Build history of the part. All positions in model axes, mm. Face numbers are marked on the shaded views. A direction names the side the tool comes from. Give positions to 0.01 mm unless a question says otherwise; leave off trailing zeros. Write each loop counter-clockwise with the first axis right and the second up, starting at its lowest first coordinate (ties: lowest second). Pieces come first, ordered by that corner, then holes. Notation, with made-up numbers: (-17, 12.5) -> (-3, 12.5) arc R13 ccw to (-3, 28.5) -> close; hole circle Ø7 at (19.5, 12.5). An arc over 180 degrees is marked (long way). Write item = value, one per line. Start each with the question number.
Q1. Saw through at C-C, the plane z = 5. List the corners of the cut face in (x, y), then the cut area to 3 significant figures.
Q2. Tool access for the marked faces 1 and 2: list every direction of +Z, -Z, +X, -X, +Y, -Y with a clear straight run to the whole face (end or side of a thin tool).
Q3. Saw through at B-B, the plane x = -2.5. List the corners of the cut face in (y, z).
Q4. Wall check: line 1 (Z direction, x = -3.5, y = -0.5); line 2 (X direction, y = -1.5, z = 7.75); line 3 (X direction, y = 5, z = 11.5). Give the ranges that are in metal, low to high.
Q5. Drop flat-ended pins along their axis: P1, Ø8, axis at x = -2, z = 7.5, coming from the +Y side; P2, Ø5, axis at y = 2, z = 6.5, coming from the -X side; P3, Ø5.5, axis at y = 3, z = 9.5, coming from the -X side; P4, Ø5.5, axis at y = 2, z = 9.5, coming from the +X side. Give the stop position or say it passes through.
Q6. Saw through at D-D, the plane x = 5.75. List the corners of the cut face in (y, z), then the cut area to 3 significant figures.
Q7. Mould opens along Y. For the marked faces 3, 4, 5 and 6 say: pulls with the +Y half, pulls with the -Y half, needs draft (parallel to the pull), parting line crosses it, or undercut.
Q8. Saw through at A-A, the plane y = 2. List the corners of the cut face in (x, z), then the cut area to 3 significant figures.
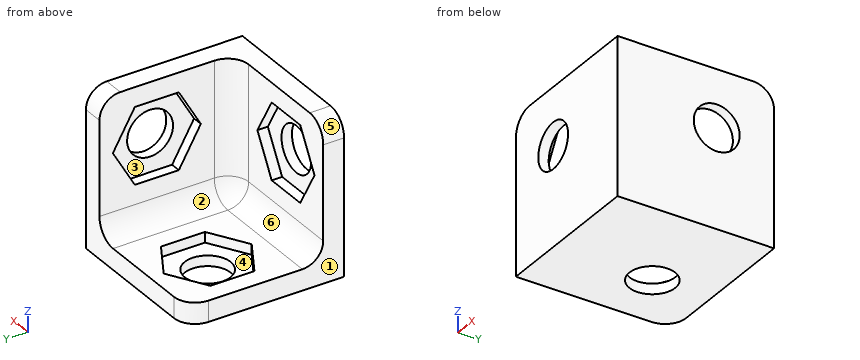
Autodesk Inventor part; units mm, degrees
ref_plane "YZ Plane" through (0, 0, 0) normal (1, 0, 0) x (0, 1, 0)
ref_plane "XZ Plane" through (0, 0, 0) normal (0, 1, 0) x (-1, 0, 0)
ref_plane "XY Plane" through (0, 0, 0) normal (0, 0, 1) x (1, 0, 0)
sketch "Sketch1" plane through (0, 0, 0) normal (0, 0, 1) x (1, 0, 0)
  line L0 (-7.5, -7.5) -> (7.5, -7.5)
  line L1 (7.5, -7.5) -> (7.5, 7.5)
  line L2 (7.5, 7.5) -> (-7.5, 7.5)
  line L3 (-7.5, 7.5) -> (-7.5, -7.5)
  line L4 (-7.5, -7.5) -> (7.5, 7.5) construction
  line L5 (7.5, -7.5) -> (-7.5, 7.5) construction
  point P0 (0, 0)
  dimension "d0" = 15
  dimension "d1" = 15
extrude "Extrusion1" add sketch "Sketch1" along normal blind 15
sketch "Sketch2" plane through (0, 0, 15) normal (0, 0, 1) x (1, 0, 0)
  line L0 (-7.5, 7.5) -> (-7.5, -7.5)
  line L1 (-7.5, 7.5) -> (5.5, 7.5)
  line L2 (5.5, 7.5) -> (5.5, -5.5)
  line L3 (5.5, -5.5) -> (-7.5, -5.5)
  line L4 (-7.5, -5.5) -> (-7.5, 7.5)
  line L5 (7.5, -7.5) -> (7.5, 7.5)
  line L6 (-7.5, -7.5) -> (7.5, -7.5)
  point P0 (0, 0)
  dimension "d4" = 2
  dimension "d5" = 2
extrude "Extrusion2" cut sketch "Sketch2" against normal blind 13
sketch "Sketch6" plane through (5.5, -5.5, 15) normal (-1, 0, 0) x (0, 0, 1)
  line L0 (-5.5, 11.7147) -> (-1.85, 9.6073)
  line L1 (-1.85, 9.6073) -> (-1.85, 5.3927)
  line L2 (-1.85, 5.3927) -> (-5.5, 3.2853)
  line L3 (-5.5, 3.2853) -> (-9.15, 5.3927)
  line L4 (-9.15, 5.3927) -> (-9.15, 9.6073)
  line L5 (-9.15, 9.6073) -> (-5.5, 11.7147)
  line L6 (0, 0) -> (-13, 0)
  line L7 (-13, 0) -> (-13, 13)
  line L8 (0, 13) -> (0, 0)
  point P0 (-15, 5.5)
  point P1 (-5.5, 7.5)
  dimension "d41" = 7.5
  dimension "d42" = 7.5
  dimension "d43" = 7.3
  dimension "d44" = 0
extrude "Extrusion3" cut sketch "Sketch6" against normal blind 1
sketch "Sketch7" plane through (6.5, -5.5, 15) normal (-1, 0, 0) x (0, 0, 1)
  circle A0 centre (-5.5, 7.5) radius 2.2
  line L0 (0, 0) -> (-13, 0)
  line L1 (-13, 0) -> (-13, 13)
  point P0 (-15, 5.5)
  dimension "d47" = 4.4
  dimension "d48" = 7.5
  dimension "d49" = 7.5
extrude "Extrusion4" cut sketch "Sketch7" against normal blind 1
sketch "Sketch8" plane through (-7.5, -5.5, 15) normal (0, 1, 0) x (1, 0, 0)
  line L0 (3.3927, 1.85) -> (1.2853, 5.5)
  line L1 (1.2853, 5.5) -> (3.3927, 9.15)
  line L2 (3.3927, 9.15) -> (7.6073, 9.15)
  line L3 (7.6073, 9.15) -> (9.7147, 5.5)
  line L4 (9.7147, 5.5) -> (7.6073, 1.85)
  line L5 (7.6073, 1.85) -> (3.3927, 1.85)
  line L6 (0, 13) -> (13, 13)
  line L7 (13, 13) -> (13, 0)
  line L8 (13, 0) -> (0, 0)
  point P0 (7.5, 15)
  point P1 (5.5, 5.5)
  dimension "d52" = 7.3
  dimension "d53" = 7.5
  dimension "d54" = 7.5
  dimension "d55" = 0
extrude "Extrusion5" cut sketch "Sketch8" against normal blind 1
sketch "Sketch9" plane through (-7.5, -6.5, 15) normal (0, 1, 0) x (1, 0, 0)
  circle A0 centre (5.5, 5.5) radius 2.2
  line L0 (0, 13) -> (13, 13)
  line L1 (0, 0) -> (0, 13)
  point P0 (7.5, 15)
  dimension "d58" = 4.4
  dimension "d59" = 7.5
  dimension "d60" = 5.5
extrude "Extrusion6" cut sketch "Sketch9" against normal blind 1
sketch "Sketch10" plane through (0, 0, 2) normal (0, 0, 1) x (1, 0, 0)
  line L0 (1.65, -0.1073) -> (-2, -2.2147)
  line L1 (-2, -2.2147) -> (-5.65, -0.1073)
  line L2 (-5.65, -0.1073) -> (-5.65, 4.1073)
  line L3 (-5.65, 4.1073) -> (-2, 6.2147)
  line L4 (-2, 6.2147) -> (1.65, 4.1073)
  line L5 (1.65, 4.1073) -> (1.65, -0.1073)
  line L6 (5.5, -5.5) -> (-7.5, -5.5)
  line L7 (5.5, 7.5) -> (5.5, -5.5)
  line L8 (-7.5, -5.5) -> (-7.5, 7.5)
  point P0 (0, 0)
  point P1 (-2, 2)
  dimension "d63" = 7.5
  dimension "d64" = 7.5
  dimension "d65" = 7.3
  dimension "d66" = 0
extrude "Extrusion7" cut sketch "Sketch10" against normal blind 1
sketch "Sketch11" plane through (0, 0, 1) normal (0, 0, 1) x (1, 0, 0)
  circle A0 centre (-2, 2) radius 2.2
  line L0 (5.5, 7.5) -> (5.5, -5.5)
  line L1 (5.5, -5.5) -> (-7.5, -5.5)
  point P0 (0, 0)
  dimension "d69" = 4.4
  dimension "d70" = 7.5
  dimension "d71" = 7.5
extrude "Extrusion8" cut sketch "Sketch11" against normal blind 1
fillet "Fillet2" radius 2 3 edges at (-1, -5.5, 2) (5.5, -5.5, 8.5) (5.5, 1, 2)
fillet "Fillet3" radius 2 3 edges at (-7.5, 7.5, 1) (6.5, 7.5, 15) (-7.5, -6.5, 15)
properties part number "23 bevestigings hoekjes 3 kanten"
Report:
q1.outline = (-7.5, -7.5) -> (7.5, -7.5) -> (7.5, 7.5) -> (5.5, 7.5) -> (5.5, -3.5) arc R2 cw to (3.5, -5.5) -> (-7.5, -5.5) -> close
q1.area = 56.9 mm2
q2.face_1 = +Z, -Z, -X, +Y, -Y
q2.face_2 = +Z, -X, +Y
q3.outline = (-7.5, 0) -> (-0.14, 0) -> (-0.14, 1) -> (-1.93, 1) -> (-1.93, 2) -> (-3.5, 2) arc R2 cw to (-5.5, 4) -> (-5.5, 5.85) -> (-6.5, 5.85) -> (-6.5, 7.36) -> (-7.5, 7.36) -> close; (-7.5, 11.64) -> (-6.5, 11.64) -> (-6.5, 13.15) -> (-5.5, 13.15) -> (-5.5, 15) -> (-7.5, 15) -> close; (4.14, 0) -> (7.5, 0) -> (7.5, 2) -> (5.93, 2) -> (5.93, 1) -> (4.14, 1) -> close
q4.line_1 = 0 to 1
q4.line_2 = 5.5 to 7.5
q4.line_3 = 6.5 to 7.5
q5.P1 = -5.44
q5.P2 = 5.5
q5.P3 = 6.5
q5.P4 = 7.5
q6.outline = (-7.5, 0) -> (7.5, 0) -> (7.5, 13) arc R2 ccw to (5.5, 15) -> (-7.5, 15) -> close; hole (-2.21, 9.5) -> (-0.11, 5.85) -> (4.11, 5.85) -> (6.21, 9.5) -> (4.11, 13.15) -> (-0.11, 13.15) -> close
q6.area = 178 mm2
q7.face_3 = undercut
q7.face_4 = undercut
q7.face_5 = needs draft
q7.face_6 = pulls with the +Y half
q8.outline = (-7.5, 0) -> (-4.2, 0) -> (-4.2, 1) -> (-5.65, 1) -> (-5.65, 2) -> (-7.5, 2) -> close; (0.2, 0) -> (7.5, 0) -> (7.5, 7.3) -> (6.5, 7.3) -> (6.5, 5.85) -> (5.5, 5.85) -> (5.5, 4) arc R2 cw to (3.5, 2) -> (1.65, 2) -> (1.65, 1) -> (0.2, 1) -> close; (5.5, 13.15) -> (6.5, 13.15) -> (6.5, 11.7) -> (7.5, 11.7) -> (7.5, 15) -> (5.5, 15) -> close
q8.area = 33.5 mm2
